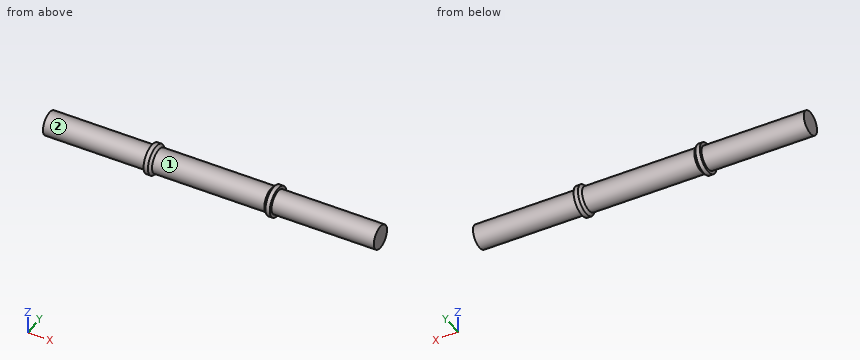
from build123d import *

# Parameters (mm, degrees)
F0_R     = 13.5
F1_DEPTH = 190
F2_R     = 17
F3_DEPTH = 72.5
F4_R     = 17.5
F4_R_2   = 14
F5_DEPTH = 67.5
F6_SIZE  = 2.99999


# Not quite as in the source:
# - a fillet or chamfer is up to 0.001 mm smaller than in the source, because OpenCascade refuses the exact size


with BuildPart() as f1:
    # F0 (on Right) → F1 (new body, symmetric)
    with BuildSketch(Plane.YZ):
        Circle(F0_R)
    extrude(amount=F1_DEPTH, both=True)

    # F2 (on Right) → F3 (join, symmetric)
    with BuildSketch(Plane.YZ):
        Circle(F2_R)
    extrude(amount=F3_DEPTH, both=True)

    # F4 (on Right) → F5 (cut, symmetric)
    with BuildSketch(Plane.YZ):
        Circle(F4_R)
        Circle(F4_R_2, mode=Mode.SUBTRACT)
    extrude(amount=F5_DEPTH, both=True, mode=Mode.SUBTRACT)

    # F6 (size 3 in the source; OpenCascade refuses exactly that, so slightly less here)
    f6_edges = [f1.edges().sort_by_distance(p)[0] for p in [
        (-67.5, -14, 0),
        (67.5, -14, 0),
    ]]
    chamfer(f6_edges, length=F6_SIZE)


solid = f1.part
Part model, mm, in its own coordinate system. Face numbers are marked on the shaded views. Give positions to 0.01 mm unless a question says otherwise; leave off trailing zeros. Loops run counter-clockwise (first coordinate to the right, second up) from the corner with the lowest first, then second, coordinate; pieces in that order, holes last. Notation, with made-up numbers: M -34,42 L 0,42 A20 ccw 0,77 Z; hole C 16.5,-36.75 d7. An arc over 180 degrees is marked long. Put each result on its own line as item: value. Start each with the question number.
1) Saw through at C-C (x = -103.5). List the corners of the cut face in (y, z).
2) Flat gauge pins, fed straight in: pin 1 (8 mm diameter, centred on x = 102, y = -6, fed in from +Z); pin 2 (8 mm diameter, centred on x = 82, z = -13.5, fed in from +Y); pin 3 (8 mm diameter, centred on x = 96.5, y = 11, fed in from -Z). Where does each tip first touch, or does it go through?
3) Saw through at D-D (x = 14.5). List the corners of the cut face in (y, z), then the cut area to 3 significant figures.
4) Pull direction X, two halves, no side cores. Call the marked faces 1 and 2: +X half, -X half, draft (parallel to the pull), parting line (faces both ways), or undercut.
5) Probe probe 1 along X at (y, z) = (11.5, -7.5); probe 2 along Y at (x, z) = (-43, 0.5); probe 3 along Y at (x, z) = (138, 0.5). List the from-to ranges inside material, lowest first.
Numbers:
1. outline: C 0,0 d27
2. pin 1: z = 13.35
2. pin 2: y = 9.59
2. pin 3: z = -11.54
3. outline: C 0,0 d28
3. area: 616 mm^2
4. face 1: undercut
4. face 2: draft
5. probe 1: -72.5 to 72.5
5. probe 2: -13.99 to 13.99
5. probe 3: -13.49 to 13.49
